from build123d import *

# Parameters (mm, degrees)
F0_W     = 12.7
F0_H     = 12.7
F1_DEPTH = 12.7
F2_R     = 3.96875
F3_DEPTH = 12.7
F4_R     = 5.4246105656
F5_DEPTH = 6.35
F6_R     = 3.175
F7_DEPTH = 3.175


# Not quite as in the source:
# - a pattern or mirror of a feature is missing from the dataset's text; its kind, count and spacing are read off the source's solid


with BuildPart() as f1:
    # F0 (on Top) → F1 (new body)
    with BuildSketch(Plane.XY):
        Rectangle(F0_W, F0_H)
    extrude(amount=F1_DEPTH)

    # F2 (on face) → F3 (cut, through all)
    with BuildSketch(Plane.XY.offset(12.7)):
        Circle(F2_R)
    extrude(amount=-F3_DEPTH, mode=Mode.SUBTRACT)

    # F4 (on face) → F5 (cut)
    with BuildSketch(Plane(origin=(0, 0, 0), x_dir=(1, 0, 0), z_dir=(0, 0, -1))):
        Circle(F4_R)
    extrude(amount=-F5_DEPTH, mode=Mode.SUBTRACT)

    # F6 (on face) → F7 (join)
    with BuildSketch(Plane.XZ.offset(6.35)):
        with Locations((0, 6.35)):
            Circle(F6_R)
    f7 = extrude(amount=F7_DEPTH)

    # F7_copies: F7 across plane
    add(f7.mirror(Plane.ZX))


solid = f1.part
Verification items for the finished model (mm, model axes). A direction names the side the tool comes from. Coordinates: 2 decimals unless noted, no trailing zeros. Order: outer loops, then holes, each group sorted by start corner. A loop starts at its lowest first (then second) coordinate and runs counter-clockwise, first axis right, second up.
1. Sectioned sample at A-A, the plane y = 0. Record the cut outline in (x, z).
Results found:
outline: (-6.35, 0) - (-5.42, 0) - (-5.42, 6.35) - (-3.97, 6.35) - (-3.97, 12.7) - (-6.35, 12.7) - close; (3.97, 6.35) - (5.42, 6.35) - (5.42, 0) - (6.35, 0) - (6.35, 12.7) - (3.97, 12.7) - close
2. Sectioned sample at D-D, the plane x = 1.5. Record the cut outline in (y, z) (3 decimals), and give its area (3 significant figures).
Results found:
outline: (-9.525, 3.552) - (-6.35, 3.552) - (-6.35, 0) - (-5.213, 0) - (-5.213, 6.35) - (-3.674, 6.35) - (-3.674, 12.7) - (-6.35, 12.7) - (-6.35, 9.148) - (-9.525, 9.148) - close; (3.674, 6.35) - (5.213, 6.35) - (5.213, 0) - (6.35, 0) - (6.35, 3.552) - (9.525, 3.552) - (9.525, 9.148) - (6.35, 9.148) - (6.35, 12.7) - (3.674, 12.7) - close
area: 84.0 mm2
3. Sectioned sample at C-C, the plane z = 4. Record the cut outline in (x, y) (3 decimals).
Results found:
outline: (-6.35, -6.35) - (-2.135, -6.35) - (-2.135, -9.525) - (2.135, -9.525) - (2.135, -6.35) - (6.35, -6.35) - (6.35, 6.35) - (2.135, 6.35) - (2.135, 9.525) - (-2.135, 9.525) - (-2.135, 6.35) - (-6.35, 6.35) - close; hole circle Ø10.849 at (0, 0)
4. Release check for a two-part mould opening along Y. For faces 1 (the face through (-3, 3, 12.7)), 2 (the face through (-0.86, -3.874, 9.569)), 3 (the face through (0, -9.525, 6)) record: +Y half, -Y half, draft (parallel to the pull), parting line (faces both ways), or undercut.
Results found:
face 1: draft
face 2: undercut
face 3: -Y half
5. Scan lines: line 1 (X direction, y = 0, z = 4.75); line 2 (Y direction, x = 0, z = 8) (3 decimals); line 3 (Y direction, x = 5.5, z = 11). Record each from-to range of solid material in increasing order.
Results found:
line 1: x = -6.35 to -5.42, 5.42 to 6.35
line 2: y = -9.525 to -3.969, 3.969 to 9.525
line 3: y = -6.35 to 6.35
6. Sectioned sample at B-B, the plane x = 0. Record the cut outline in (y, z) (3 decimals), and give its area (3 significant figures).
Results found:
outline: (-9.525, 3.175) - (-6.35, 3.175) - (-6.35, 0) - (-5.425, 0) - (-5.425, 6.35) - (-3.969, 6.35) - (-3.969, 12.7) - (-6.35, 12.7) - (-6.35, 9.525) - (-9.525, 9.525) - close; (3.969, 6.35) - (5.425, 6.35) - (5.425, 0) - (6.35, 0) - (6.35, 3.175) - (9.525, 3.175) - (9.525, 9.525) - (6.35, 9.525) - (6.35, 12.7) - (3.969, 12.7) - close
area: 82.3 mm2
7. Set-up check for faces 4 (the face through (-4.305, 3.301, 3.131)), 5 (the face through (1.707, -7.915, 9.027)), 6 (the face through (-2, 6.35, 3)): record each of +Z, -Z, +X, -X, +Y, -Y from which the full face is reachable in a straight line by a thin tool's end or side.
Results found:
face 4: -Z
face 5: -Y
face 6: +Y
8. Go/stop test with flat-tipped pins: pin 1 Ø1 at (x, z) = (3.5, 10.5) entering from -Y; pin 2 Ø1.5 at (x, y) = (-3.5, -7.5) entering from -Z. Record where each tip stops, or that it passes through.
Results found:
pin 1: stops at y = -6.35
pin 2: stops at z = 4.76
